Check sheet for the modelled part. Datum: model origin and axes. Units: mm. A direction names the side the tool comes from. Round coordinates to 2 decimals unless told otherwise and drop trailing zeros. Write each loop counter-clockwise with the first axis right and the second up, starting at its lowest first coordinate (ties: lowest second). Pieces come first, ordered by that corner, then holes. Notation, with made-up numbers: (19.25, 83) - (45.25, 83) arc R18 ccw to (45.25, 113) - close; hole circle Ø11 at (-12.5, 78.5). An arc over 180 degrees is marked (long way). Use one line per item in the form item = value. Start each with the question number.
1) Section check A-A (z = 0). Record the boundary of the cut face in (x, y), then the cut area to 4 significant figures.
2) Gauge pin test, flat ends, axial feed: P1, Ø1.5, axis at x = -4, y = -23.5, coming from the +Z side; P2, Ø4, axis at x = -4, z = 1, coming from the -Y side; P3, Ø5, axis at x = 2.5, y = -22.5, coming from the +Z side; P4, Ø1, axis at x = 1, y = 15.5, coming from the +Z side. Record the tip position at first contact, or that the pin passes through.
3) Scan lines: probe 1 along Z at (x, y) = (-0.25, -30); probe 2 along Y at (x, z) = (3, -1.5); probe 3 along X at (y, z) = (-4, -0.25). Record each from-to range of solid material in increasing order.
4) Section check B-B (x = 0). Record the boundary of the cut face in (y, z), then the cut area to 4 significant figures.
5) Set-up check for faces 1 (the face through (0, -33, 0)), 2 (the face through (-2, -19, -2)), 3 (the face through (-2.44, 25.84, -0.54)): record each of +Z, -Z, +X, -X, +Y, -Y from which the full face is reachable in a straight line by a thin tool's end or side.
6) Section check D-D (y = -24.5). Record the boundary of the cut face in (x, z).
7) Section check C-C (y = 2.5). Record the boundary of the cut face in (x, z), then the cut area to 3 significant figures.
from build123d import *

# Parameters (mm, degrees)
CHAMFER_SIZE = 0.5


with BuildPart() as part:
    # Sketch → Revolution (revolve)
    with BuildSketch(Plane.YZ):
        Polygon((-33, 0), (-33, 2.5), (-19, 2.5), (-19, 5), (19, 5), (19, 2.5), (33, 2.5), (33, 0), align=None)
    revolve(axis=Axis((0, 0, 0), (0, 1, 0)))

    # Chamfer
    chamfer_edges = [part.edges().sort_by_distance(p)[0] for p in [
        (0, 33, -2.5),
        (0, -33, -2.5),
    ]]
    chamfer(chamfer_edges, length=CHAMFER_SIZE)


solid = part.part
Results are:
q1.outline = (-5, -19) - (-2.5, -19) - (-2.5, -32.5) - (-2, -33) - (2, -33) - (2.5, -32.5) - (2.5, -19) - (5, -19) - (5, 19) - (2.5, 19) - (2.5, 32.5) - (2, 33) - (-2, 33) - (-2.5, 32.5) - (-2.5, 19) - (-5, 19) - close
q1.area = 519.5 mm²
q2.P1 = through
q2.P2 = -32.88
q2.P3 = 2.5
q2.P4 = 4.97
q3.probe_1 = -2.49 to 2.49
q3.probe_2 = -19 to 19
q3.probe_3 = -4.99 to 4.99
q4.outline = (-33, -2) - (-32.5, -2.5) - (-19, -2.5) - (-19, -5) - (19, -5) - (19, -2.5) - (32.5, -2.5) - (33, -2) - (33, 2) - (32.5, 2.5) - (19, 2.5) - (19, 5) - (-19, 5) - (-19, 2.5) - (-32.5, 2.5) - (-33, 2) - close
q4.area = 519.5 mm²
q5.face_1 = +Z, -Z, +X, -X, -Y
q5.face_2 = -Y
q5.face_3 = +Y
q6.outline = circle Ø5 at (0, 0)
q7.outline = circle Ø10 at (0, 0)
q7.area = 78.5 mm²
